Can you work these out from the model? Positions are in its coordinate system, mm. Round coordinates to 2 decimals unless told otherwise and drop trailing zeros. Order: outer loops, then holes, each group sorted by start corner. A loop starts at its lowest first (then second) coordinate and runs counter-clockwise, first axis right, second up. Notation, with made-up numbers: M -25,-13.5 L 34,-13.5 A11 cw 34,7.5 Z; hole C 42.25,12 d6. An arc over 180 degrees is marked long. One line per question, with ' | ' between items.
```python
from build123d import *

# Parameters (mm, degrees)
F1_DEPTH = 60
F2_SIZE  = 1.5


with BuildPart() as f1:
    # F0 (on Front) → F1 (new body)
    with BuildSketch(Plane.XZ):
        Polygon((-57.5, 24.006124), (-57.5, -9.314226), (41, -9.314226), (41, 24.006124), (37.5, 24.006124), (37.5, -7.686828), (21, -7.686828), (21, 24.006124), (17.5, 24.006124), (17.5, -7.764603), (9, -7.764603), (9, 24.006124), (5.5, 24.006124), (5.5, -7.764603), (0, -7.764603), (0, 24.006124), (-3.5, 24.006124), (-3.5, -7.764603), (-9, -7.764603), (-9, 24.006124), (-12.5, 24.006124), (-12.5, -7.764603), (-18, -7.764603), (-18, 24.006124), (-21.5, 24.006124), (-21.5, -7.764603), (-29, -7.764603), (-29, 24.006124), (-32.5, 24.006124), (-32.5, -7.764603), (-45, -7.764603), (-45, 24.006124), (-48.5, 24.006124), (-48.5, -7.764603), (-54, -7.764603), (-54, 24.006124), align=None)
    extrude(amount=F1_DEPTH)

    # F2
    f2_edges = [f1.edges().sort_by_distance(p)[0] for p in [
        (37.5, -30, 24.006124),
        (21, -30, 24.006124),
        (17.5, -30, 24.006124),
        (9, -30, 24.006124),
        (5.5, -30, 24.006124),
        (0, -30, 24.006124),
        (-3.5, -30, 24.006124),
        (-9, -30, 24.006124),
        (-12.5, -30, 24.006124),
        (-18, -30, 24.006124),
        (-21.5, -30, 24.006124),
        (-29, -30, 24.006124),
        (-32.5, -30, 24.006124),
        (-45, -30, 24.006124),
        (-48.5, -30, 24.006124),
        (-54, -30, 24.006124),
        (9, -60, 8.120761),
        (5.5, -60, 8.120761),
        (37.5, -60, 8.159648),
        (21, -60, 8.159648),
        (17.5, -60, 8.120761),
        (0, -60, 8.120761),
        (-3.5, -60, 8.120761),
        (-12.5, -60, 8.120761),
        (-18, -60, 8.120761),
        (-21.5, -60, 8.120761),
        (-29, -60, 8.120761),
        (-32.5, -60, 8.120761),
        (-45, -60, 8.120761),
        (-48.5, -60, 8.120761),
        (-54, -60, 8.120761),
        (-9, -60, 8.120761),
    ]]
    chamfer(f2_edges, length=F2_SIZE)


solid = f1.part
```
(1) Thinking about a two-plate mould opening in X: for faces 1 (the flat face through (29, -30, -7.687)), 2 (the flat face through (40, -30, 24.006)), 3 (the flat face through (-57.5, -30, 8)), which applies, released by +X, released by -X, zero draft, split by the parting line, or undercut?
Final values:
face 1: undercut | face 2: zero draft | face 3: released by -X
(2) If we section it at B-B on x = -40: Please give me the cut outline in (y, z).
Final values:
outline: M -60,-9.31 L 0,-9.31 L 0,-7.76 L -60,-7.76 Z
(3) If we section it at A-A on z = 21: State how many separate pieces and enclosed holes the cut face has, plus the area to 3 significant figures.
Final values:
separate pieces: 9 | enclosed holes: 0 | area: 1,870 mm^2
(4) Please list where these lines run through material, in increasing order: probe 1 along Z at (x, y) = (-17, -53); probe 2 along Z at (x, y) = (34, -46); probe 3 along Y at (x, z) = (-11.5, 2.5). Write a range as [from, to].
Final values:
probe 1: [-9.31, -7.76] | probe 2: [-9.31, -7.69] | probe 3: [-59.5, 0]
(5) If we section it at C-C on x = 29: Please give me the cut outline in (y, z).
Final values:
outline: M -60,-9.31 L 0,-9.31 L 0,-7.69 L -60,-7.69 Z
(6) Will these pins go through, and if not, where does the flat tip stop? pin 1 Ø12.5 at (x, y) = (-40.5, -42) entering from +Z; pin 2 Ø3.5 at (x, y) = (10.5, -21) entering from +Z; pin 3 Ø2.5 at (x, y) = (-14.5, -31) entering from +Z; pin 4 Ø1.5 at (x, z) = (-43, 2) entering from -Y.
Final values:
pin 1: z = 24.01 | pin 2: z = 22.76 | pin 3: z = -7.76 | pin 4: through
